```python
from build123d import *

# Parameters (mm, degrees)
F1_DEPTH = 8
F2_R     = 5


with BuildPart() as f1:
    # F0 (on Front) → F1 (new body)
    with BuildSketch(Plane.XZ):
        Polygon((-4.7884929424, 6.975), (-35, 6.975), (-35, -6.975), (-4.7552655505, -6.975), align=None)
        with BuildLine():
            Line((-4.815391477, 18.2679283934), (-4.7884929424, 6.975))
            Line((-4.7884929424, 6.975), (4.7552655505, 6.975))
            Line((4.7552655505, 6.975), (4.7226697487, 20.6598368154))
            ThreePointArc((4.7226697487, 20.6598368154), (0.0998647972, 18.880787826), (-4.815391477, 18.2679283934))
        make_face()
        Polygon((4.7552655505, 6.975), (-4.7884929424, 6.975), (-4.7552655505, -6.975), (4.7884929424, -6.975), align=None)
        Polygon((35, 6.975), (4.7552655505, 6.975), (4.7884929424, -6.975), (35, -6.975), align=None)
        with BuildLine():
            ThreePointArc((-24.048441977, 31.7176597434), (-16.5588212007, 21.9513310022), (-4.815391477, 18.2679283934))
            Line((-4.815391477, 18.2679283934), (-4.863998607, 38.674870505))
            ThreePointArc((-4.863998607, 38.674870505), (-13.5241307894, 32.6260370701), (-24.048441977, 31.7176597434))
        make_face()
        with BuildLine():
            add(Edge.make_bspline(
                [(-13.1900259225, 24.8776112918), (-13.3247436315, 25.0045940128), (-13.3247436315, 25.2946560658)],
                knots=[0, 0, 0, 1, 1, 1], degree=2))
            add(Edge.make_bspline(
                [(-13.3247436315, 25.2946560658), (-13.3247436315, 25.5653806485), (-13.2016284046, 25.7039658516)],
                knots=[0, 0, 0, 1, 1, 1], degree=2))
            add(Edge.make_bspline(
                [(-13.2016284046, 25.7039658516), (-13.0785131777, 25.8425510547), (-12.8490418647, 25.8425510547)],
                knots=[0, 0, 0, 1, 1, 1], degree=2))
            add(Edge.make_bspline(
                [(-12.8490418647, 25.8425510547), (-12.6157030576, 25.8425510547), (-12.4848528426, 25.7039658516)],
                knots=[0, 0, 0, 1, 1, 1], degree=2))
            add(Edge.make_bspline(
                [(-12.4848528426, 25.7039658516), (-12.3540026276, 25.5653806485), (-12.3540026276, 25.2946560658)],
                knots=[0, 0, 0, 1, 1, 1], degree=2))
            add(Edge.make_bspline(
                [(-12.3540026276, 25.2946560658), (-12.3540026276, 25.0329556358), (-12.4867865897, 24.8917921033)],
                knots=[0, 0, 0, 1, 1, 1], degree=2))
            add(Edge.make_bspline(
                [(-12.4867865897, 24.8917921033), (-12.6195705517, 24.7506285709), (-12.8490418647, 24.7506285709)],
                knots=[0, 0, 0, 1, 1, 1], degree=2))
            add(Edge.make_bspline(
                [(-12.8490418647, 24.7506285709), (-13.0553082135, 24.7506285709), (-13.1900259225, 24.8776112918)],
                knots=[0, 0, 0, 1, 1, 1], degree=2))
        make_face(mode=Mode.SUBTRACT)
        with BuildLine():
            Line((-16.0190978123, 26.9705701495), (-14.6732098866, 30.7581359787))
            Line((-14.6732098866, 30.7581359787), (-13.9370968544, 30.7581359787))
            Line((-13.9370968544, 30.7581359787), (-16.0590619174, 24.8679425567))
            Line((-16.0590619174, 24.8679425567), (-16.7358733743, 24.8679425567))
            Line((-16.7358733743, 24.8679425567), (-18.8475251198, 30.7581359787))
            Line((-18.8475251198, 30.7581359787), (-18.1217254051, 30.7581359787))
            Line((-18.1217254051, 30.7581359787), (-16.7681024913, 26.9473651853))
            add(Edge.make_bspline(
                [(-16.7681024913, 26.9473651853), (-16.5347636842, 26.2898911986), (-16.3981122282, 25.6698029876)],
                knots=[0, 0, 0, 1, 1, 1], degree=2))
            add(Edge.make_bspline(
                [(-16.3981122282, 25.6698029876), (-16.2524366193, 26.3221203156), (-16.0190978123, 26.9705701495)],
                knots=[0, 0, 0, 1, 1, 1], degree=2))
        make_face(mode=Mode.SUBTRACT)
        with BuildLine():
            Line((-9.0176444363, 27.3173554484), (-10.2475075409, 27.3173554484))
            Line((-10.2475075409, 27.3173554484), (-10.2475075409, 24.8679425567))
            Line((-10.2475075409, 24.8679425567), (-10.9320539858, 24.8679425567))
            Line((-10.9320539858, 24.8679425567), (-10.9320539858, 30.7581359787))
            Line((-10.9320539858, 30.7581359787), (-9.316730642, 30.7581359787))
            add(Edge.make_bspline(
                [(-9.316730642, 30.7581359787), (-8.2325431463, 30.7581359787), (-7.7149435274, 30.3430249518)],
                knots=[0, 0, 0, 1, 1, 1], degree=2))
            add(Edge.make_bspline(
                [(-7.7149435274, 30.3430249518), (-7.1973439085, 29.9279139249), (-7.1973439085, 29.0938243771)],
                knots=[0, 0, 0, 1, 1, 1], degree=2))
            add(Edge.make_bspline(
                [(-7.1973439085, 29.0938243771), (-7.1973439085, 27.9258411772), (-8.3820862492, 27.5145976444)],
                knots=[0, 0, 0, 1, 1, 1], degree=2))
            Line((-8.3820862492, 27.5145976444), (-6.7822328816, 24.8679425567))
            Line((-6.7822328816, 24.8679425567), (-7.5918283005, 24.8679425567))
            Line((-7.5918283005, 24.8679425567), (-9.0176444363, 27.3173554484))
        make_face(mode=Mode.SUBTRACT)
        with BuildLine():
            Line((-4.863998607, 38.674870505), (-4.815391477, 18.2679283934))
            ThreePointArc((-4.815391477, 18.2679283934), (0.0998647972, 18.880787826), (4.7226697487, 20.6598368154))
            Line((4.7226697487, 20.6598368154), (4.7060632326, 27.6318224688))
            Line((4.7060632326, 27.6318224688), (4.6783778732, 39.2550869399))
            Line((4.6783778732, 39.2550869399), (-4.863998607, 38.674870505))
        make_face()
        with BuildLine():
            Line((4.7060632326, 27.6318224688), (4.7226697487, 20.6598368154))
            ThreePointArc((4.7226697487, 20.6598368154), (7.9719953336, 22.8103532241), (10.7533443371, 25.5392605699))
            ThreePointArc((10.7533443371, 25.5392605699), (7.6471719178, 26.3470332103), (4.7060632326, 27.6318224688))
        make_face()
        with BuildLine():
            ThreePointArc((-24.048441977, 31.7176597434), (-13.5241307894, 32.6260370701), (-4.863998607, 38.674870505))
            ThreePointArc((-4.863998607, 38.674870505), (-14.4325081161, 43.1503482577), (-20.481341551, 51.8104804401))
            ThreePointArc((-20.481341551, 51.8104804401), (-24.9568193037, 42.241970931), (-24.048441977, 31.7176597434))
        make_face()
        with BuildLine():
            ThreePointArc((-36.0986844951, 64.9460903753), (-39.6657849211, 44.8532696785), (-24.048441977, 31.7176597434))
            ThreePointArc((-24.048441977, 31.7176597434), (-24.9568193037, 42.241970931), (-20.481341551, 51.8104804401))
            ThreePointArc((-20.481341551, 51.8104804401), (-30.0498510602, 56.2859581928), (-36.0986844951, 64.9460903753))
        make_face()
        with BuildLine():
            Line((4.6783778732, 39.2550869399), (4.7060632326, 27.6318224688))
            ThreePointArc((4.7060632326, 27.6318224688), (7.6471719178, 26.3470332103), (10.7533443371, 25.5392605699))
            ThreePointArc((10.7533443371, 25.5392605699), (15.2288220897, 35.107770079), (14.3204447631, 45.6320812666))
            ThreePointArc((14.3204447631, 45.6320812666), (9.9604022486, 41.7465620958), (4.6783778732, 39.2550869399))
        make_face()
        with BuildLine():
            ThreePointArc((14.3204447631, 45.6320812666), (15.2288220897, 35.107770079), (10.7533443371, 25.5392605699))
            ThreePointArc((10.7533443371, 25.5392605699), (29.9377877071, 32.4964713315), (33.5048881331, 52.5892920282))
            ThreePointArc((33.5048881331, 52.5892920282), (24.8447559507, 46.5404585933), (14.3204447631, 45.6320812666))
        make_face()
        with BuildLine():
            ThreePointArc((-36.0986844951, 64.9460903753), (-30.0498510602, 56.2859581928), (-20.481341551, 51.8104804401))
            ThreePointArc((-20.481341551, 51.8104804401), (-21.3897188777, 62.3347916277), (-16.914241125, 71.9033011369))
            ThreePointArc((-16.914241125, 71.9033011369), (-27.4385523126, 70.9949238102), (-36.0986844951, 64.9460903753))
        make_face()
        with BuildLine():
            ThreePointArc((-13.347140699, 91.9961218336), (-32.5315840691, 85.038911072), (-36.0986844951, 64.9460903753))
            ThreePointArc((-36.0986844951, 64.9460903753), (-27.4385523126, 70.9949238102), (-16.914241125, 71.9033011369))
            ThreePointArc((-16.914241125, 71.9033011369), (-17.8226184517, 82.4276123244), (-13.347140699, 91.9961218336))
        make_face()
        with BuildLine():
            ThreePointArc((17.8875451891, 65.7249019633), (18.7959225157, 55.2005907757), (14.3204447631, 45.6320812666))
            ThreePointArc((14.3204447631, 45.6320812666), (24.8447559507, 46.5404585933), (33.5048881331, 52.5892920282))
            ThreePointArc((33.5048881331, 52.5892920282), (27.4560546982, 61.2494242106), (17.8875451891, 65.7249019633))
        make_face()
        with BuildLine():
            ThreePointArc((17.8875451891, 65.7249019633), (27.4560546982, 61.2494242106), (33.5048881331, 52.5892920282))
            ThreePointArc((33.5048881331, 52.5892920282), (37.0719885591, 72.6821127249), (21.4546456151, 85.81772266))
            ThreePointArc((21.4546456151, 85.81772266), (22.3630229418, 75.2934114724), (17.8875451891, 65.7249019633))
        make_face()
        with BuildLine():
            ThreePointArc((-13.347140699, 91.9961218336), (-17.8226184517, 82.4276123244), (-16.914241125, 71.9033011369))
            ThreePointArc((-16.914241125, 71.9033011369), (-10.710686982, 76.8736634045), (-3.078749577, 79.0967505652))
            ThreePointArc((-3.078749577, 79.0967505652), (-5.2212274005, 83.0794109578), (-3.4549967043, 87.2426097465))
            ThreePointArc((-3.4549967043, 87.2426097465), (-8.0755153119, 90.296848239), (-13.347140699, 91.9961218336))
        make_face()
        with BuildLine():
            ThreePointArc((2.6166495696, 78.7959161107), (11.9730736035, 74.2710294822), (17.8875451891, 65.7249019633))
            ThreePointArc((17.8875451891, 65.7249019633), (22.3630229418, 75.2934114724), (21.4546456151, 85.81772266))
            ThreePointArc((21.4546456151, 85.81772266), (12.6866425633, 85.4580279417), (4.880367051, 81.4493722528))
            ThreePointArc((4.880367051, 81.4493722528), (3.9763704464, 79.9282503523), (2.6166495696, 78.7959161107))
        make_face()
        with BuildLine():
            ThreePointArc((21.4546456151, 85.81772266), (5.837302671, 98.9533325952), (-13.347140699, 91.9961218336))
            ThreePointArc((-13.347140699, 91.9961218336), (-8.0755153119, 90.296848239), (-3.4549967043, 87.2426097465))
            ThreePointArc((-3.4549967043, 87.2426097465), (2.1518386227, 88.0838664996), (5.2267939203, 83.3205729723))
            ThreePointArc((5.2267939203, 83.3205729723), (5.1394575354, 82.3690736675), (4.880367051, 81.4493722528))
            ThreePointArc((4.880367051, 81.4493722528), (12.6866425633, 85.4580279417), (21.4546456151, 85.81772266))
        make_face()
    extrude(amount=F1_DEPTH)

    # F2
    f2_edges = [f1.edges().sort_by_distance(p)[0] for p in [
        (-19.894246, -8, 6.975),
        (-35, -8, 0),
        (0, -8, -6.975),
        (35, -8, 0),
        (19.877633, -8, 6.975),
    ]]
    fillet(f2_edges, radius=F2_R)


solid = f1.part
```
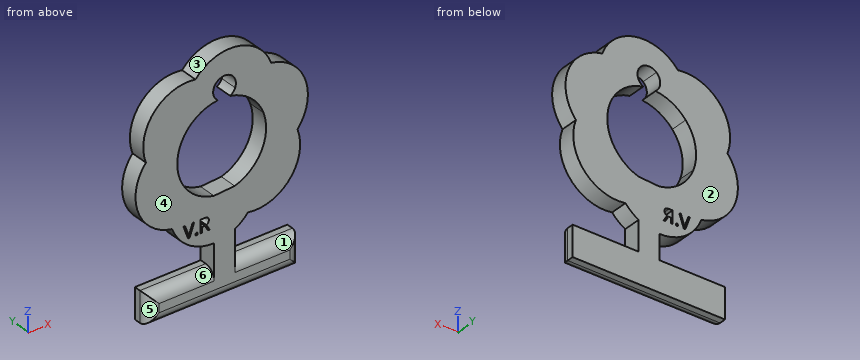
Model file for the job. Use its own axes, mm. Face numbers are marked on the shaded views. A direction names the side the tool comes from. Give positions to 0.01 mm unless a question says otherwise; leave off trailing zeros. Order: outer loops, then holes, each group sorted by start corner. A loop starts at its lowest first (then second) coordinate and runs counter-clockwise, first axis right, second up.
1) Pin check, flat tips, straight feed: pin 1 (1.4 mm diameter, centred on x = -9.5, y = -3, fed in from +Z); pin 2 (2 mm diameter, centred on y = -7, z = 50, fed in from -X); pin 3 (0.9 mm diameter, centred on y = -2, z = -3, fed in from -X). Stop position of each tip, or through.
2) Saw through at C-C, the plane z = 5. Write the cut outline in (x, y) (3 decimals), then the cut area to 3 significant figures.
3) Wall check: probe 1 along Z at (x, y) = (14, -6) (3 decimals); probe 2 along Z at (x, y) = (9.5, -7) (3 decimals); probe 3 along Z at (x, y) = (26, -2.25) (3 decimals). Give the ranges that are in metal, low to high.
4) Saw through at A-A, the plane z = 76. Write the cut outline in (x, y), then the cut area to 3 significant figures.
5) Saw through at D-D, the plane z = 90.5. Write the cut outline in (x, y).
6) 3-axis set-ups, long thin cutter, end or side, ignore diameter. For the marked faces 4, 5 and 6: which of +Z, -Z, +X, -X, +Y, -Y reach the whole face in a straight line?
7) Mould opens along Z. For the marked faces 1, 2 and 3 say: +Z half, -Z half, draft (parallel to the pull), parting line (faces both ways), or undercut.
8) Saw through at B-B, the plane y = -4.75. Count the separate pieces of the cut face and the enclosed holes in it, then the cut area to 3 significant figures.
Computed:
1. pin 1: stops at z = 96
1. pin 2: stops at x = -40.87
1. pin 3: stops at x = -35
2. outline: (-35, -3) arc R5 ccw to (-33.025, -6.981) - (-4.784, -6.981) - (-4.784, -8) - (4.76, -8) - (4.76, -6.981) - (33.025, -6.981) arc R5 ccw to (35, -3) - (35, 0) - (-35, 0) - close
2. area: 494 mm2
3. probe 1: z = -5.975 to 5.975, 25.228 to 45.26, 72.275 to 95.56
3. probe 2: z = -4.975 to 4.975, 24.179 to 41.451, 76.085 to 97.944
3. probe 3: z = -6.975 to 6.975, 28.898 to 84.45
4. outline: (-36.91, -8) - (-12.23, -8) - (-12.23, 0) - (-36.91, 0) - close; (9.63, -8) - (35.52, -8) - (35.52, 0) - (9.63, 0) - close
4. area: 404 mm2
5. outline: (-25.32, -8) - (19.03, -8) - (19.03, 0) - (-25.32, 0) - close
6. face 4: +Z, -Z, +X, -X, -Y
6. face 5: -Z, -X, -Y
6. face 6: -X, -Y
7. face 1: undercut
7. face 2: draft
7. face 3: +Z half
8. separate pieces: 1
8. enclosed holes: 4
8. area: 4,410 mm2
